Can you work these out from the drawing? Everything is in mm from the part's minimum corner. A direction names the side the tool comes from. Round coordinates to 2 decimals unless told otherwise and drop trailing zeros. Order: outer loops, then holes, each group sorted by start corner. A loop starts at its lowest first (then second) coordinate and runs counter-clockwise, first axis right, second up. Notation, with made-up numbers: M 73.25,42.5 L 97.25,42.5 A14 cw 97.25,46.5 Z; hole C 27.5,47.25 d2. An arc over 180 degrees is marked long. Use one line per item in the form item = value. Start each with the question number.
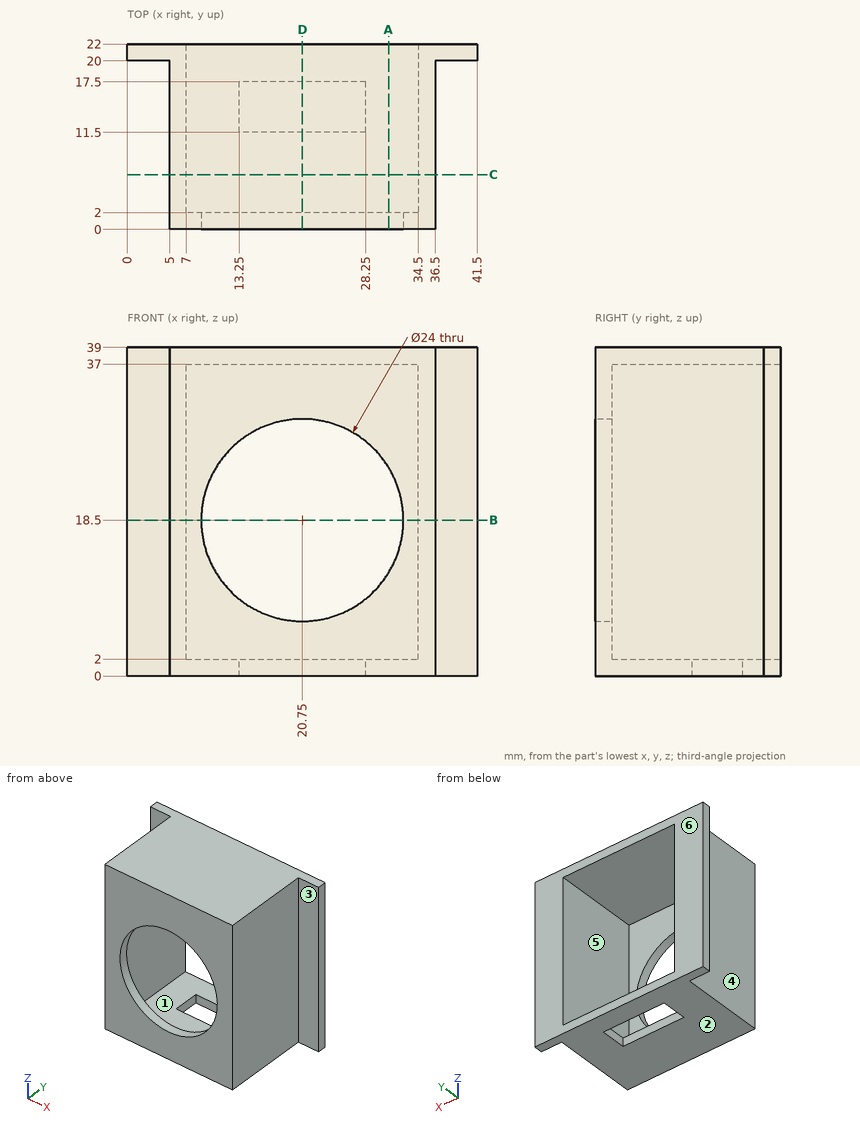
1) Will these pins go through, and if not, where does the flat tip stop? pin 1 Ø6 at (y, z) = (10, 27) entering from +X; pin 2 Ø10 at (y, z) = (10, 26) entering from -X; pin 3 Ø10 at (x, z) = (28.5, 7.5) entering from +Y.
2) If we section it at A-A on x = 31: Write out the boundary of the cut face in (y, z).
3) If we section it at D-D on x = 20.75: Write out the boundary of the cut face in (y, z).
4) If we mould it in two halves opening along X, with no side actions, what happens to the marked faces 4, 5 and 6? For each: +X half, -X half, draft (parallel to the pull), parting line (faces both ways), or undercut.
5) If we section it at C-C on y = 6.5: Write out the boundary of the cut face in (x, z), then the cut area to 3 significant figures.
6) If we section it at B-B on z = 18.5: Write out the boundary of the cut face in (x, y).
7) On a 3-axis mill with a long thin cutter (end or side, diameter ignored), from which of +Z, -Z, +X, -X, +Y, -Y can I reach the whole of each face in a straight line? I mean the marked faces 1, 2 and 3. Say none if no direction works.
8) If I drill on line 1 (X direction, y = 1.2, z = 18.5); line 2 (X direction, y = 13.5, z = 4.5); line 3 (Z direction, x = 8, y = 14), over which ranges is the centre line in solid material (lowest first)?
Completed:
q1.pin_1 = 36.5
q1.pin_2 = 5
q1.pin_3 = 2
q2.outline = M 0,0 L 22,0 L 22,2 L 2,2 L 2,12.26 L 0,12.26 Z; M 0,24.74 L 2,24.74 L 2,37 L 22,37 L 22,39 L 0,39 Z
q3.outline = M 0,0 L 11.5,0 L 11.5,2 L 2,2 L 2,6.5 L 0,6.5 Z; M 0,30.5 L 2,30.5 L 2,37 L 22,37 L 22,39 L 0,39 Z; M 17.5,0 L 22,0 L 22,2 L 17.5,2 Z
q4.face_4 = -X half
q4.face_5 = undercut
q4.face_6 = draft
q5.outline = M 5,0 L 36.5,0 L 36.5,39 L 5,39 Z; hole M 7,2 L 34.5,2 L 34.5,37 L 7,37 Z
q5.area = 266 mm²
q6.outline = M 0,20 L 5,20 L 5,0 L 8.75,0 L 8.75,2 L 7,2 L 7,22 L 0,22 Z; M 32.75,0 L 36.5,0 L 36.5,20 L 41.5,20 L 41.5,22 L 34.5,22 L 34.5,2 L 32.75,2 Z
q7.face_1 = +Y
q7.face_2 = -Z, +X, -X, +Y, -Y
q7.face_3 = +Z, -Z, +X, -Y
q8.line_1 = 5 to 8.75, 32.75 to 36.5
q8.line_2 = 5 to 7, 34.5 to 36.5
q8.line_3 = 0 to 2, 37 to 39
